from build123d import *

# Parameters (mm, degrees)
F1_ANGLE = 180
F3_DEPTH = 38.1
F4_ANGLE = 60
F8_COUNT = 5


with BuildPart() as f1:
    # F0 (on Top) → F1 (revolve)
    with BuildSketch(Plane.XY):
        with BuildLine():
            Line((0, 0), (0, -25.4))
            ThreePointArc((0, -25.4), (25.4, 0), (0, 25.4))
            Line((0, 25.4), (0, 0))
        make_face()
    revolve(axis=Axis((0, -19.9486762285, 0), (0, -1, 0)), revolution_arc=F1_ANGLE)


with BuildPart() as f3:
    # F2 (on face) → F3 (new body)
    with BuildSketch(Plane(origin=(0, 0, 0), x_dir=(1, 0, 0), z_dir=(0, 0, -1))):
        with BuildLine():
            Line((0, -6.9453125), (0, 6.9453125))
            ThreePointArc((0, 6.9453125), (-6.9453125, 0), (0, -6.9453125))
        make_face()
        with BuildLine():
            ThreePointArc((0, -6.9453125), (4.9110775662, -4.9110775662), (6.9453125, 0))
            ThreePointArc((6.9453125, 0), (4.9110775662, 4.9110775662), (0, 6.9453125))
            Line((0, 6.9453125), (0, -6.9453125))
        make_face()
    extrude(amount=-F3_DEPTH)


with BuildPart() as f4_1:
    # F4: copy of F3
    add(f3.part.rotate(Axis((0, 0.6129407927, 0), (0, -1, 0)), F4_ANGLE))


with BuildPart() as f4_1_1:
    # F7: moved
    add(f4_1.part.moved(Location((-10.9985226281, 0, 6.35))))


with BuildPart() as f8_1:
    # F8: instance of F4_1
    add(f4_1_1.part.rotate(Axis((0, 0, 10.6922788545), (0, 0, -1)), 1 * 360 / F8_COUNT))


with BuildPart() as f8_2:
    # F8: instance of F4_1
    add(f4_1_1.part.rotate(Axis((0, 0, 10.6922788545), (0, 0, -1)), 2 * 360 / F8_COUNT))


with BuildPart() as f8_3:
    # F8: instance of F4_1
    add(f4_1_1.part.rotate(Axis((0, 0, 10.6922788545), (0, 0, -1)), 3 * 360 / F8_COUNT))


with BuildPart() as f8_4:
    # F8: instance of F4_1
    add(f4_1_1.part.rotate(Axis((0, 0, 10.6922788545), (0, 0, -1)), 4 * 360 / F8_COUNT))


with BuildPart() as f1_1:
    add(f1.part)

    # F9: cut F8_1, F8_2, F8_3, F8_4, F4_1, F3
    add(f8_1.part, mode=Mode.SUBTRACT)
    add(f8_2.part, mode=Mode.SUBTRACT)
    add(f8_3.part, mode=Mode.SUBTRACT)
    add(f8_4.part, mode=Mode.SUBTRACT)
    add(f4_1_1.part, mode=Mode.SUBTRACT)
    add(f3.part, mode=Mode.SUBTRACT)


solid = f1_1.part
The listing builds one solid part. Answer for the finished solid, in the listing's coordinates (mm). Round coordinates to 2 decimals unless told otherwise and drop trailing zeros. Use a Markdown table: item, result. Add a question column.
1. Consider line 1 (Y direction, x = 10.5, z = 10.5); line 2 (Y direction, x = 12, z = 9); line 3 (Z direction, x = -12.5, y = -3). Determine where each line is inside the solid, lowest interval first.
2. Flat-ended cylindrical pins translate along their axes: P1, Ø2, axis at x = -16.5, z = 6, coming from the +Y side; P2, Ø3, axis at x = -2.5, z = 18, coming from the +Y side; P3, Ø1, axis at x = 5.5, z = 19.5, coming from the -Y side. Find the tip coordinate at first contact, or state that the pin passes through.
3. The part is cut by section A-A (y = 2). Give the number of separate pieces and of enclosed holes in the cut face, and give its area (3 significant figures).
4. For a pull along Y with two mould halves and no side action, classify faces 1 (the face through (-11.047, -0.097, 6.266)), 2 (the face through (5.3, -5.3, 0)) as +Y half, -Y half, draft (parallel to the pull), parting line (faces both ways), or undercut.
Reported:
| question | item | result |
|---|---|---|
| 1 | line 1 | -20.61 to -16.21, -1.11 to 1.11, 16.21 to 20.61 |
| 1 | line 2 | -20.5 to -16.93, -0.81 to 0.81, 16.93 to 20.5 |
| 1 | line 3 | 0 to 3.75, 14.45 to 21.91 |
| 2 | P1 | y = 19.26 |
| 2 | P2 | y = 18.93 |
| 2 | P3 | y = -15.96 |
| 3 | separate pieces | 2 |
| 3 | enclosed holes | 1 |
| 3 | area | 488 mm^2 |
| 4 | face 1 | undercut |
| 4 | face 2 | draft |
